For this review, take the finished solid that the model builds, in its own axes (mm). Face numbers are marked on the shaded views. A direction names the side the tool comes from. Coordinates: 2 decimals unless noted, no trailing zeros. Write each loop counter-clockwise with the first axis right and the second up, starting at its lowest first coordinate (ties: lowest second). Pieces come first, ordered by that corner, then holes. Notation, with made-up numbers: (8.25, 30.25) -> (63.25, 30.25) arc R16 cw to (63.25, 35.25) -> close; hole circle Ø9 at (68.5, -34.5). An arc over 180 degrees is marked (long way). One line per item, written item: value. Start each with the question number.
1) For probe 1 along Y at (x, z) = (0, 18.25); probe 2 along Z at (x, y) = (9.5, 22); probe 3 along Z at (x, y) = (-26, 15), list the stretches that pass through material, from the lowest coordinate up. Write a range as from..to.
2) Add section A-A (z = 5). State the section outline as (x, y) points, and give its area (3 significant figures).
3) Add section B-B (z = -40). State the section outline as (x, y) points.
4) Machinability: for the marked faces 1 and 2, which of the approach directions +Z, -Z, +X, -X, +Y, -Y give a long, thin tool a straight path to every point of the face, cutting with its end or side? Answer none if there is none.
5) Add section C-C (z = 31.5). State the section outline as (x, y) points, and give its area (3 significant figures).
6) For pin 1 Ø5 at (x, z) = (20, 39) entering from -Y; pin 2 Ø8 at (y, z) = (9, 35) entering from +X; pin 3 Ø6 at (x, z) = (-32.5, 15) entering from +Y, all flat-tipped, find the tip position at first contact; note any pin that passes through.
7) Mouldability with a two-part tool opening along Y and no side actions: class the marked faces 3, 4 and 5 as released by +Y, released by -Y, zero draft, split by the parting line, or undercut.
from build123d import *

# Parameters (mm, degrees)
F3_R = 5.08
F4_R = 5.08
F5_R = 5.08


# Not quite as in the source:
# - a fillet or chamfer that OpenCascade refuses, or shapes differently, is made with other operations: its cross-section is extruded or revolved along the edge and cut away or added


with BuildPart() as f1:
    # F0 (on Front) → F1 (revolve)
    with BuildSketch(Plane.XZ):
        Polygon((-31.5286010422, 51.7711788416), (-32.5126800885, 53.8890883327), (-32.7099710703, 53.8890883327), (-41.6522659361, 36.9457937777), (-41.6522659361, 7.7656768262), (-32.7099710703, -6.3537354581), (-12.7074699849, -6.3537354581), (-4.7064702958, -6.3537354581), (-4.7064702958, -65.6552687287), (-9.4129405916, -68.7144696712), (-29.415441677, -68.7144696712), (-29.415441677, -72.4796503782), (0, -72.4796503782), (0, -4.3968333285), (-12.472147122, -4.3968333285), (-31.5333530307, -4.3968333285), (-39.5343527198, 8.2363234833), (-39.5343527198, 36.475148052), (-31.5333530307, 51.7711788416), align=None)
    revolve(axis=Axis((0, 0, -0.3529824317), (0, 0, -1)))

    # F2: fillet of radius 7.62 on 1 edges, made by hand

    # F2_s1 → F2_t2 (revolve, cut)
    with BuildSketch(Plane.XZ):
        with BuildLine():
            ThreePointArc((-32.5126800885, 53.8890883327), (-33.0044959985, 53.2373184877), (-33.4237493814, 52.5366663478))
            Line((-33.4237493814, 52.5366663478), (-32.7099710703, 53.8890883327))
            Line((-32.7099710703, 53.8890883327), (-32.5126800885, 53.8890883327))
        make_face()
    revolve(axis=Axis((0, 0, 53.8890883327), (0, 0, -1)), mode=Mode.SUBTRACT)

    # F3
    f3_edges = [f1.edges().sort_by_distance(p)[0] for p in [
        (41.652266, 0, 36.945794),
    ]]
    fillet(f3_edges, radius=F3_R)

    # F4
    f4_edges = [f1.edges().sort_by_distance(p)[0] for p in [
        (41.652266, 0, 7.765677),
    ]]
    fillet(f4_edges, radius=F4_R)

    # F5
    f5_edges = [f1.edges().sort_by_distance(p)[0] for p in [
        (32.709971, 0, -6.353735),
    ]]
    fillet(f5_edges, radius=F5_R)


solid = f1.part
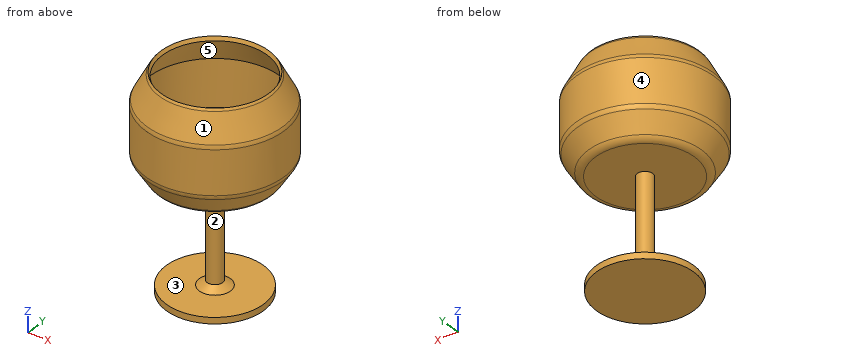
Numbers:
1. probe 1: -41.65..-39.53, 39.53..41.65
1. probe 2: -72.48..-68.71, -6.35..-4.4
1. probe 3: -6.35..-4.4
2. outline: circle Ø79.8 at (0, 0); hole circle Ø74.97 at (0, 0)
2. area: 587 mm²
3. outline: circle Ø9.41 at (0, 0)
4. face 1: +Z
4. face 2: none
5. outline: circle Ø83.3 at (0, 0); hole circle Ø79.07 at (0, 0)
5. area: 540 mm²
6. pin 1: y = -37.19
6. pin 2: x = 41.35
6. pin 3: y = 29.41
7. face 3: zero draft
7. face 4: split by the parting line
7. face 5: undercut
